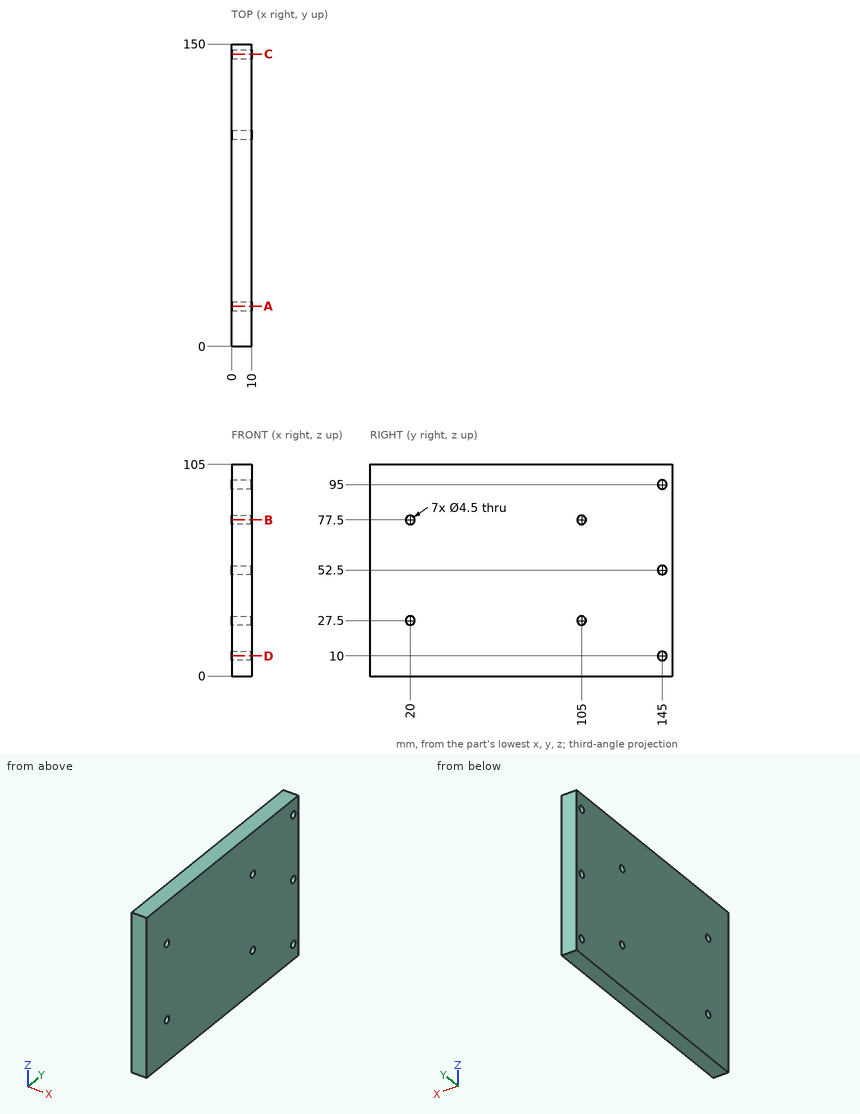
Print and shaded views of the part. All mm, measured from the part's lowest x, y and z. Round coordinates to 2 decimals unless told otherwise and drop trailing zeros. Write each loop counter-clockwise with the first axis right and the second up, starting at its lowest first coordinate (ties: lowest second). Pieces come first, ordered by that corner, then holes. Notation, with made-up numbers: (46, 31) - (93, 31) arc R26 cw to (93, 51) - close; hole circle Ø6 at (-39.75, 62.25). An arc over 180 degrees is marked (long way). One line per question, with ' | ' between items.
1. Drill centre lines: line 1 along Y through (x, z) = (6.25, 77.5); line 2 along Z through (x, y) = (6.25, 145); line 3 along Y through (x, z) = (4.25, 52.5). Where is each one in solid material? Low to high. Write a range as from..to.
Results are:
line 1: 0..17.75, 22.25..102.75, 107.25..150 | line 2: 0..7.75, 12.25..50.25, 54.75..92.75, 97.25..105 | line 3: 0..142.75, 147.25..150
2. Band-saw the part on C-C, the plane y = 145. Write the cut outline in (x, z).
Results are:
outline: (0, 0) - (10, 0) - (10, 7.75) - (0, 7.75) - close; (0, 12.25) - (10, 12.25) - (10, 50.25) - (0, 50.25) - close; (0, 54.75) - (10, 54.75) - (10, 92.75) - (0, 92.75) - close; (0, 97.25) - (10, 97.25) - (10, 105) - (0, 105) - close
3. Band-saw the part on A-A, the plane y = 20. Write the cut outline in (x, z), and give its area (3 significant figures).
Results are:
outline: (0, 0) - (10, 0) - (10, 25.25) - (0, 25.25) - close; (0, 29.75) - (10, 29.75) - (10, 75.25) - (0, 75.25) - close; (0, 79.75) - (10, 79.75) - (10, 105) - (0, 105) - close | area: 960 mm^2
4. Band-saw the part on B-B, the plane z = 77.5. Write the cut outline in (x, y), and give its area (3 significant figures).
Results are:
outline: (0, 0) - (10, 0) - (10, 17.75) - (0, 17.75) - close; (0, 22.25) - (10, 22.25) - (10, 102.75) - (0, 102.75) - close; (0, 107.25) - (10, 107.25) - (10, 150) - (0, 150) - close | area: 1,410 mm^2
5. Band-saw the part on D-D, the plane z = 10. Write the cut outline in (x, y).
Results are:
outline: (0, 0) - (10, 0) - (10, 142.75) - (0, 142.75) - close; (0, 147.25) - (10, 147.25) - (10, 150) - (0, 150) - close
